from build123d import *

# Parameters (mm, degrees)
BOSS_EXTRUDE1_DEPTH = 57.5


with BuildPart() as part:
    # Sketch1 → Boss-Extrude1 (new, symmetric)
    with BuildSketch(Plane.XY):
        Polygon((0, 0), (0, 21), (90, 21), (90, 0), (86.5, 0), (86.5, 11), (61.5, 11), (61.5, 16), (28.5, 16), (28.5, 11), (3.5, 11), (3.5, 0), align=None)
    extrude(amount=BOSS_EXTRUDE1_DEPTH, both=True)


solid = part.part
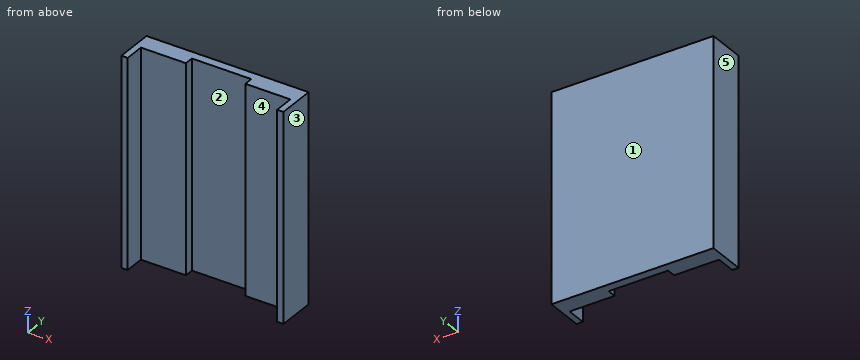
Can you work these out from the model? Positions are in its coordinate system, mm. Face numbers are marked on the shaded views. A direction names the side the tool comes from. Coordinates: 2 decimals unless noted, no trailing zeros. Loops run counter-clockwise (first coordinate to the right, second up) from the corner with the lowest first, then second, coordinate; pieces in that order, holes last. Notation, with made-up numbers: (28, 61) - (57, 61) arc R32 cw to (57, 96) - close; hole circle Ø7 at (36, 41). An arc over 180 degrees is marked (long way). Answer as a JSON object with one key per item and string values. Group by question number.
Item 1: On a 3-axis mill with a long thin cutter (end or side, diameter ignored), from which of +Z, -Z, +X, -X, +Y, -Y can I reach the whole of each face in a straight line? I mean the marked faces 1 and 2. Say none if no direction works.
Item 2: If we section it at C-C (x = 67.5): List the corners of the cut face in (y, z) for me, plus the area to 3 significant figures.
Item 3: If we section it at A-A (y = 3): List the corners of the cut face in (x, z) for me, plus the area to 3 significant figures.
Item 4: If we section it at B-B (z = 37): List the corners of the cut face in (x, y) for me.
Item 5: If we mould it in two halves opening along X, with no side actions, what happens to the marked faces 3, 4 and 5? For each: released by +X, released by -X, zero draft, split by the parting line, or undercut.
Item 6: If I drill on L1, parallel to X at y = 6.75, z = -33; L2, parallel to X at y = 15.5, z = 6; L3, parallel to Y at x = 47, z = 16.5, over which ranges is the centre line in solid material (lowest first)? Write a range as from..to.
Item 7: For pin 1 (20 mm diameter, centred on x = 79, z = 15, fed in from -Y); pin 2 (5 mm diameter, centred on x = 38.5, z = 40, fed in from -Y); pin 3 (7.5 mm diameter, centred on x = 11, z = -23.5, fed in from -Y), each with a flat end and sliding along its axis, tell me the tip position at first contact or that it passes through.
Item 8: If we section it at D-D (x = 37.5): List the corners of the cut face in (y, z) for me.
Returned:
{
 "1": {"face 1": "+Z, -Z, +X, -X, +Y", "face 2": "+Z, -Z, -Y"},
 "2": {"outline": "(11, -57.5) - (21, -57.5) - (21, 57.5) - (11, 57.5) - close", "area": "1,150 mm²"},
 "3": {"outline": "(0, -57.5) - (3.5, -57.5) - (3.5, 57.5) - (0, 57.5) - close; (86.5, -57.5) - (90, -57.5) - (90, 57.5) - (86.5, 57.5) - close", "area": "805 mm²"},
 "4": {"outline": "(0, 0) - (3.5, 0) - (3.5, 11) - (28.5, 11) - (28.5, 16) - (61.5, 16) - (61.5, 11) - (86.5, 11) - (86.5, 0) - (90, 0) - (90, 21) - (0, 21) - close"},
 "5": {"face 3": "released by +X", "face 4": "undercut", "face 5": "released by -X"},
 "6": {"L1": "x = 0..3.5, 86.5..90", "L2": "x = 0..28.5, 61.5..90", "L3": "y = 16..21"},
 "7": {"pin 1": "stops at y = 0", "pin 2": "stops at y = 16", "pin 3": "stops at y = 11"},
 "8": {"outline": "(16, -57.5) - (21, -57.5) - (21, 57.5) - (16, 57.5) - close"}
}
